from build123d import *

# Parameters (mm, degrees)
EXTRUDE_1_DEPTH     = 10
SKETCH_2_R          = 10
EXTRUDE_2_DEPTH     = 15
SKETCH_3_W          = 24
SKETCH_3_H          = 4
CUT_EXTRUDE_1_DEPTH = 61
SKETCH_4_R          = 5
CUT_EXTRUDE_2_DEPTH = 23
EXTRUDE_3_DEPTH     = 22
EXTRUDE_4_DEPTH     = 3
EXTRUDE_START       = 8
SKETCH_7_R          = 23
EXTRUDE_5_DEPTH     = 30
SKETCH_9_R          = 17.5
EXTRUDE_6_DEPTH     = 10
SKETCH_10_R         = 10
CUT_EXTRUDE_3_DEPTH = 15
SKETCH_12_R         = 17
CUT_EXTRUDE_4_DEPTH = 3
SKETCH_13_R         = 15
CUT_EXTRUDE_5_DEPTH = 22


with BuildPart() as part:
    # 草图1 → 凸台-拉伸1 (new body)
    with BuildSketch(Plane(origin=(0, 0, 0), x_dir=(1, 0, 0), z_dir=(0, 1, 0))):
        with BuildLine():
            Line((-14.5, 30.5), (14.5, 30.5))
            ThreePointArc((14.5, 30.5), (20.156854249, 28.156854249), (22.5, 22.5))
            Line((22.5, 22.5), (22.5, -22.5))
            ThreePointArc((22.5, -22.5), (20.156854249, -28.156854249), (14.5, -30.5))
            Line((14.5, -30.5), (-14.5, -30.5))
            ThreePointArc((-14.5, -30.5), (-20.156854249, -28.156854249), (-22.5, -22.5))
            Line((-22.5, -22.5), (-22.5, 22.5))
            ThreePointArc((-22.5, 22.5), (-20.156854249, 28.156854249), (-14.5, 30.5))
        make_face()
    extrude(amount=-EXTRUDE_1_DEPTH)

    # 草图2 → 凸台-拉伸2 (add)
    with BuildSketch(Plane(origin=(0, 0, 0), x_dir=(1, 0, 0), z_dir=(0, 1, 0))):
        with Locations(Location((0, 0, 0), (0, 0, 270))):
            Circle(SKETCH_2_R)
    extrude(amount=EXTRUDE_2_DEPTH)

    # 草图3 → 切除-拉伸1 (cut)
    with BuildSketch(Plane.XY.offset(30.5)):
        with Locations((0, -10)):
            Rectangle(SKETCH_3_W, SKETCH_3_H)
    extrude(amount=-CUT_EXTRUDE_1_DEPTH, mode=Mode.SUBTRACT)

    # 草图4 → 切除-拉伸2 (cut)
    with BuildSketch(Plane(origin=(0, 15, 0), x_dir=(1, 0, 0), z_dir=(0, 1, 0))):
        with Locations(Location((0, 0, 0), (0, 0, 270))):
            Circle(SKETCH_4_R)
    extrude(amount=-CUT_EXTRUDE_2_DEPTH, mode=Mode.SUBTRACT)

    # 草图6 → 凸台-拉伸3 (add, symmetric)
    with BuildSketch(Plane.XY):
        with BuildLine():
            Line((22.5, -8), (67, -8))
            ThreePointArc((67, -8), (71.242640687, -6.242640687), (73, -2))
            Line((73, -2), (73, 40))
            Line((73, 40), (67, 40))
            Line((67, 40), (67, -2))
            Line((67, -2), (22.5, -2))
            Line((22.5, -2), (22.5, -8))
        make_face()
    extrude(amount=EXTRUDE_3_DEPTH, both=True)

    # 草图6<3> → 凸台-拉伸4 (add, symmetric)
    with BuildSketch(Plane.XY):
        with BuildLine():
            ThreePointArc((35, 10), (40.656854249, 12.343145751), (43, 18))
            Line((43, 18), (43, 40))
            Line((43, 40), (67, 40))
            Line((67, 40), (67, -2))
            Line((67, -2), (22.5, -2))
            Line((22.5, -2), (6.5, -2))
            Line((6.5, -2), (6.5, 10))
            Line((6.5, 10), (35, 10))
        make_face()
    extrude(amount=EXTRUDE_4_DEPTH, both=True)

    # 草图7 → 凸台-拉伸5 (add)
    with BuildSketch(Plane(origin=(73, 0, 0), x_dir=(0, 0, -1), z_dir=(1, 0, 0)).offset(EXTRUDE_START)):
        with Locations((0, 40)):
            Circle(SKETCH_7_R)
    extrude(amount=-EXTRUDE_5_DEPTH)

    # 草图9 → 凸台-拉伸6 (add)
    with BuildSketch(Plane.ZY.offset(-51)):
        with Locations(Location((0, 40, 0), (0, 0, 260.129110394))):
            Circle(SKETCH_9_R)
    extrude(amount=EXTRUDE_6_DEPTH)

    # 草图10 → 切除-拉伸3 (cut)
    with BuildSketch(Plane.ZY.offset(-41)):
        with Locations((0, 40)):
            Circle(SKETCH_10_R)
    extrude(amount=-CUT_EXTRUDE_3_DEPTH, mode=Mode.SUBTRACT)

    # 草图12 → 切除-拉伸4 (cut)
    with BuildSketch(Plane.ZY.offset(-56)):
        with Locations((0, 40)):
            Circle(SKETCH_12_R)
    extrude(amount=-CUT_EXTRUDE_4_DEPTH, mode=Mode.SUBTRACT)

    # 草图13 → 切除-拉伸5 (cut)
    with BuildSketch(Plane.ZY.offset(-59)):
        with Locations((0, 40)):
            Circle(SKETCH_13_R)
    extrude(amount=-CUT_EXTRUDE_5_DEPTH, mode=Mode.SUBTRACT)


solid = part.part
Source: CAD feature listing. Evaluate the final solid. Frame: model axes, mm. A direction names the side the tool comes from. Round coordinates to 2 decimals unless told otherwise and drop trailing zeros. Loops run counter-clockwise (first coordinate to the right, second up) from the corner with the lowest first, then second, coordinate; pieces in that order, holes last.
Q1. Section A-A, the plane x = 0. Return loops of the section in (y, z), plus the area to 3 significant figures.
Q2. Access query for faces 1 (the face through (55, -4, -22)), 2 (the face through (40.594, 12.281, 0.042)), 3 (the face through (55, -4, 22)), 4 (the face through (57.479, 23.404, -3.685)), 5 (the face through (67, 12, -12)). Directions: +Z, -Z, +X, -X, +Y, -Y. A direction counts if a zero-diameter tool reaches every point of the face in a straight line with its end or side. Return the directions, or none.
Q3. Section C-C, the plane z = 0. State how many separate pieces and enclosed holes the cut face has, plus the area to 3 significant figures.
Q4. Ray query, line 1 (Y direction, x = 57.35, z = 0); line 2 (X direction, y = 49, z = -8.5); line 3 (X direction, y = 3, z = 11.5). Return the intervals inside material, ascending.
Q5. Section B-B, the plane y = 40. Return loops of the section in (x, z).
Q6. Mould query, pull axis Y, two halves, no side actions, for faces 6 (the face through (51, 48.7, 15.4)), 7 (the face through (81, 25, -5)), 8 (the face through (-17, -10, 0)), 9 (the face through (46.07, 55.507, -8.11)). Classes: pulls with the +Y half, pulls with the -Y half, needs draft (parallel to the pull), parting line crosses it, or undercut.
Q7. Section D-D, the plane y = 27. Return loops of the section in (x, z), plus the area to 3 significant figures.
Q8. First-contact query: P1, Ø16, axis at x = -1.5, z = -3.5, coming from the +Y side; P2, Ø5.5, axis at y = 15, z = 10.5, coming from the -X side; P3, Ø10, axis at y = 51, z = 11.5, coming from the -X side. Flat tips, straight axial feed; report the tip coordinate or a pass-through.
Solutions:
1. outline: (-8, -30.5) - (0, -30.5) - (0, -10) - (15, -10) - (15, -5) - (-8, -5) - close; (-8, 5) - (15, 5) - (15, 10) - (0, 10) - (0, 30.5) - (-8, 30.5) - close
1. area: 558 mm2
2. face 1: -Z, +X, -Y
2. face 2: +Z, -Z
2. face 3: +Z, +X, -Y
2. face 4: none
2. face 5: -Z
3. separate pieces: 3
3. enclosed holes: 0
3. area: 2,430 mm2
4. line 1: y = -8 to 23, 57 to 63
4. line 2: x = 41 to 56
4. line 3: x = 67 to 73
5. outline: (41, -17.5) - (51, -17.5) - (51, -23) - (81, -23) - (81, -15) - (59, -15) - (59, -17) - (56, -17) - (56, -10) - (41, -10) - close; (41, 10) - (56, 10) - (56, 17) - (59, 17) - (59, 15) - (81, 15) - (81, 23) - (51, 23) - (51, 17.5) - (41, 17.5) - close
6. face 6: undercut
6. face 7: needs draft
6. face 8: pulls with the -Y half
6. face 9: undercut
7. outline: (41, -11.72) - (51, -11.72) - (51, -18.97) - (67, -18.97) - (67, -22) - (73, -22) - (73, -18.97) - (81, -18.97) - (81, -7.48) - (59, -7.48) - (59, -10.95) - (56, -10.95) - (56, 10.95) - (59, 10.95) - (59, 7.48) - (81, 7.48) - (81, 18.97) - (73, 18.97) - (73, 22) - (67, 22) - (67, 18.97) - (51, 18.97) - (51, 11.72) - (41, 11.72) - close
7. area: 1,010 mm2
8. P1: stops at y = 15
8. P2: stops at x = -6.32
8. P3: stops at x = 41
